Design review of the part built by this model. Coordinates are the model's own, in mm. A direction names the side the tool comes from. Round coordinates to 2 decimals unless told otherwise and drop trailing zeros. Order: outer loops, then holes, each group sorted by start corner. A loop starts at its lowest first (then second) coordinate and runs counter-clockwise, first axis right, second up. Notation, with made-up numbers: (-7.5, -17.75) - (14.5, -17.75) arc R25 ccw to (14.5, 10.25) - close; hole circle Ø8 at (9, 65). An arc over 180 degrees is marked (long way). Write item = value, one per line.
Autodesk Inventor part; units mm, degrees
ref_plane "YZ Plane" through (0, 0, 0) normal (1, 0, 0) x (0, 1, 0)
ref_plane "XZ Plane" through (0, 0, 0) normal (0, 1, 0) x (-1, 0, 0)
ref_plane "XY Plane" through (0, 0, 0) normal (0, 0, 1) x (1, 0, 0)
sketch "Boceto1" plane through (0, 0, 0) normal (0, 1, 0) x (-1, 0, 0)
  line L0 (100, 80) -> (-100, 80)
  line L1 (-100, 80) -> (-100, -80)
  line L2 (-100, -80) -> (100, -80)
  line L3 (100, -80) -> (100, 80)
  line L4 (100, 80) -> (-100, -80) construction
  line L5 (-100, 80) -> (100, -80) construction
  point P0 (0, 0)
  dimension "d0" = 200
  dimension "d1" = 160
extrude "Extrusión1" add sketch "Boceto1" along normal blind 20
sketch "Boceto2" plane through (0, 20, 0) normal (0, 1, 0) x (1, 0, 0)
  line L0 (-100, 80) -> (-100, -80)
  line L1 (-100, 80) -> (-70, 80)
  line L2 (-70, 80) -> (-70, 40)
  line L3 (-70, 40) -> (-100, 40)
  line L4 (-100, 40) -> (-100, 80)
  line L5 (100, 80) -> (-100, 80)
  line L6 (0, 80) -> (0, 40)
  line L7 (100, 80) -> (70, 80)
  line L8 (70, 80) -> (70, 40)
  line L9 (70, 40) -> (100, 40)
  line L10 (100, 40) -> (100, 80)
  point P0 (0, 0)
  dimension "d4" = 30
  dimension "d5" = 40
extrude "Extrusión2" cut sketch "Boceto2" against normal blind 10
sketch "Boceto3" plane through (0, 20, 0) normal (0, 1, 0) x (1, 0, 0)
  line L0 (-70, 80) -> (-70, 40)
  line L1 (-70, 80.0001) -> (-70, 40)
  line L2 (-70, 40) -> (-100, 40)
  line L3 (-100, 40) -> (-100, 80.0001)
  line L4 (-100, 40) -> (-70, 40)
  line L5 (-70, 40) -> (-70, 80)
  line L6 (-70, 80) -> (-100, 80)
  line L7 (-100, 80) -> (-100, 40)
  circle A0 centre (-88.25, 58.25) radius 1.75
  circle A1 centre (-81.75, 51.75) radius 1.75
  line L8 (100, 80) -> (-100, 80)
  line L9 (0, 80) -> (0, 56.5)
  circle A2 centre (88.25, 58.25) radius 1.75
  circle A3 centre (81.75, 51.75) radius 1.75
  point P0 (0, 0)
  point P1 (-64.3507, 80)
  point P2 (-74.3507, 0)
  point P3 (-85, 80)
  dimension "d23" = 21.75
  dimension "d24" = 11.75
  dimension "d26" = 11.75
hole "Agujero1" at (-81.75, 20, -51.75) at (-88.25, 20, -58.25) at (81.75, 20, -51.75) at (88.25, 20, -58.25) direction (0, -1, 0) diameter 3.5 end through all
sketch "Boceto4" plane through (-100, 0, 80) normal (0, 0, 1) x (1, 0, 0)
  line L0 (30, 20) -> (60, 20)
  line L1 (60, 20) -> (60, 10)
  line L2 (60, 10) -> (30, 10)
  line L3 (30, 10) -> (30, 20)
  line L4 (0, 0) -> (0, 20)
  line L5 (100, 0) -> (100, 10)
  line L6 (170, 20) -> (140, 20)
  line L7 (140, 20) -> (140, 10)
  line L8 (140, 10) -> (170, 10)
  line L9 (170, 10) -> (170, 20)
  dimension "d34" = 30
  dimension "d35" = 10
  dimension "d36" = 30
extrude "Extrusión3" add sketch "Boceto4" along normal blind 40
sketch "Boceto5" plane through (0, 20, 0) normal (0, 1, 0) x (1, 0, 0)
  line L0 (59.9999, -50) -> (69.9999, -50)
  line L1 (49.9999, -101.75) -> (49.9999, -79.9497)
  line L2 (59.9999, -108.25) -> (59.9999, -50)
  line L3 (40, -80) -> (69.9999, -80)
  line L4 (49.9999, -79.9497) -> (40, -80)
  circle A0 centre (51.7499, -101.75) radius 1.75
  circle A1 centre (58.2499, -108.25) radius 1.75
  line L5 (69.9999, -80) -> (69.9999, -120)
  line L6 (40, -120) -> (40, -80)
  line L7 (69.9999, -120) -> (40, -120)
  line L8 (0, -50) -> (0, -71.75)
  line L9 (-40, -120) -> (-40, -80)
  line L10 (-49.9999, -101.75) -> (-49.9999, -79.9497)
  circle A2 centre (-51.7499, -101.75) radius 1.75
  circle A3 centre (-58.2499, -108.25) radius 1.75
  line L11 (-40, -80) -> (-69.9999, -80)
  line L12 (-69.9999, -120) -> (-40, -120)
  line L13 (-69.9999, -80) -> (-69.9999, -120)
  line L14 (-59.9999, -108.25) -> (-59.9999, -50)
  line L15 (-40, -120) -> (-69.9999, -120)
  line L16 (-69.9999, -80) -> (-69.9999, -120)
  line L17 (-40, -120) -> (-70, -120)
  line L18 (-40, -80) -> (-40, -120)
  line L19 (-59.9999, -110) -> (-49.9999, -110)
  line L20 (-49.9999, -110) -> (-49.9999, -100)
  line L21 (-49.9999, -100) -> (-59.9999, -100)
  line L22 (-59.9999, -100) -> (-59.9999, -110)
  line L23 (-100, 40) -> (-100, -80)
  point P0 (0, 0)
  point P1 (-56.75, -68.25)
  point P2 (-63.25, -61.75)
  point P3 (63.25, -61.75)
  point P4 (56.75, -68.25)
  dimension "d45" = 3.5
  dimension "d46" = 3.5
  dimension "d39" = 10
  dimension "d40" = 10
  dimension "d41" = 40
  dimension "d42" = 0
  dimension "d43" = 6.5
  dimension "d44" = 6.5
  dimension "d47" = 11.7499
  dimension "d48" = 11.75
  dimension "d49" = 0
  dimension "d50" = 11.75
  dimension "d51" = 0
  dimension "d97" = 40.0001
hole "Agujero2" at (-58.2499, 20, 108.25) at (-51.7499, 20, 101.75) at (51.7499, 20, 101.75) at (58.2499, 20, 108.25) direction (0, -1, 0) diameter 3.5 end through all
sketch "Boceto6" plane through (0, 20, 0) normal (0, 1, 0) x (1, 0, 0)
  circle A0 centre (-60.569, -13.1067) radius 10
  circle A1 centre (-29.569, -59.1067) radius 3.5
  line L0 (-60.569, -13.1067) -> (-39.0083, -13.1067)
  circle A2 centre (-29.569, 25.8933) radius 3.5
  circle A3 centre (-88.569, 25.8933) radius 3.5
  circle A4 centre (-88.569, -59.1067) radius 3.5
  line L1 (70.4544, -63.0517) -> (18.4544, -63.0517)
  line L2 (18.4544, -63.0517) -> (18.4544, 6.9483)
  line L3 (18.4544, 6.9483) -> (70.4544, 6.9483)
  line L4 (70.4544, 6.9483) -> (70.4544, -63.0517)
  line L5 (70.4544, 6.9483) -> (48.4544, 6.9483)
  line L6 (48.4544, 6.9483) -> (48.4544, 48.9483)
  line L7 (48.4544, 48.9483) -> (70.4544, 48.9483)
  line L8 (70.4544, 48.9483) -> (70.4544, 6.9483)
  line L9 (77.2288, -8.158) -> (77.2281, -5.6604)
  circle A5 centre (63.7706, -5.7606) radius 1.75
  line L10 (70.7641, -24.1464) -> (70.7641, 22.2796)
  circle A6 centre (35.8307, -5.7609) radius 1.75
  line L11 (25.1581, -13.2381) -> (25.1581, -10.7404)
  circle A7 centre (68.8507, -57.8309) radius 1.75
  line L12 (26.4277, 35.0051) -> (26.4277, 37.5029)
  circle A8 centre (20.6074, -56.5614) radius 1.75
  line L13 (18.6941, -55.9176) -> (70.7641, -55.9176)
  line L14 (18.6941, -55.9176) -> (18.6941, -7.6743)
  line L15 (44.7291, -55.9176) -> (44.7291, -31.7959)
  line L16 (63.7706, -28.0517) -> (26.4277, -28.0517)
  line L17 (44.7291, -23.5247) -> (44.7291, -31.7959)
  point P0 (0, 0)
  point P1 (-60.569, -16.6067)
  point P2 (45.425, 12.8886)
  point P3 (44.7291, -28.0517)
  dimension "d59" = 7
  dimension "d60" = 7
  dimension "d61" = 7
  dimension "d62" = 39
  dimension "d63" = 46
  dimension "d64" = 59
  dimension "d65" = 46
  dimension "d66" = 39
  dimension "d67" = 59
  dimension "d68" = 52
  dimension "d69" = 70
  dimension "d70" = 22
  dimension "d71" = 42
  dimension "d72" = 3.5
  dimension "d73" = 3.5
  dimension "d74" = 3.5
  dimension "d75" = 3.5
  dimension "d142" = 17.3763
  dimension "d143" = 12.7092
  dimension "d144" = 6.6837
  dimension "d145" = 12.7089
  dimension "d146" = 5.2208
  dimension "d147" = 1.6037
  dimension "d148" = 2.1531
  dimension "d149" = 6.4903
hole "Agujero3" at (68.8507, 20, 57.8309) at (20.6074, 20, 56.5614) at (63.7706, 20, 5.7606) at (35.8307, 20, 5.7609) direction (0, -1, 0) diameter 3.5 end through all
sketch "Boceto7" plane through (0, 20, 0) normal (0, 1, 0) x (1, 0, 0)
  circle A0 centre (-60.569, -13.1067) radius 10
  circle A1 centre (-29.569, -59.1067) radius 3.5
  line L0 (-60.569, -13.1067) -> (-39.0083, -13.1067)
  circle A2 centre (-29.569, 25.8933) radius 3.5
  circle A3 centre (-88.569, 25.8933) radius 3.5
  circle A4 centre (-88.569, -59.1067) radius 3.5
  point P0 (0, 0)
  point P1 (-60.569, -16.6067)
  dimension "d83" = 7
  dimension "d84" = 7
  dimension "d85" = 7
  dimension "d86" = 39
  dimension "d87" = 46
  dimension "d88" = 59
  dimension "d89" = 46
  dimension "d90" = 39
  dimension "d91" = 59
extrude "Extrusión4" cut sketch "Boceto7" against normal blind 20
ref_plane "Plano de trabajo1" through (0, 0, -80) normal (-1, 0, 0) x (0, 0, 1)
ref_plane "Plano de trabajo2" through (100, 0, 0) normal (0, 0, -1) x (-1, 0, 0)
sketch "Boceto8" plane through (0, 20, 0) normal (0, 1, 0) x (1, 0, 0)
  line L0 (80, -15) -> (90, -15)
  circle A0 centre (85, -10) radius 1.75
  line L1 (85, 10) -> (85, -10)
  line L2 (90, -15) -> (90, 15)
  circle A1 centre (85, 10) radius 1.75
  line L3 (80, 15) -> (80, -15)
  line L4 (90, 15) -> (80, -15) construction
  line L5 (80, 15) -> (90, -15) construction
  line L6 (90, 15) -> (80, 15)
  line L7 (100, -80) -> (100, 40)
  line L8 (0, 0) -> (20, -20)
  line L9 (0, 0) -> (28.2843, 0) construction
  line L10 (15, -60) -> (15, -70)
  circle A2 centre (10, -65) radius 1.75
  line L11 (-10, -65) -> (10, -65)
  line L12 (15, -70) -> (-15, -70)
  circle A3 centre (-10, -65) radius 1.75
  line L13 (-15, -60) -> (15, -60)
  line L14 (-15, -70) -> (15, -60) construction
  line L15 (-15, -60) -> (15, -70) construction
  line L16 (-15, -70) -> (-15, -60)
  line L17 (0, 0) -> (18.6615, 18.6615)
  line L18 (0, 0) -> (26.3913, 0) construction
  line L19 (-15, 60) -> (-15, 70)
  circle A4 centre (-10, 65) radius 1.75
  line L20 (10, 65) -> (-10, 65)
  line L21 (-15, 70) -> (15, 70)
  circle A5 centre (10, 65) radius 1.75
  line L22 (15, 60) -> (-15, 60)
  line L23 (15, 70) -> (-15, 60) construction
  line L24 (15, 60) -> (-15, 70) construction
  line L25 (15, 70) -> (15, 60)
  line L26 (70, 80) -> (-70, 80)
  line L27 (-40, -80) -> (40, -80)
  point P0 (86.9608, 0)
  point P1 (86.9608, 0)
  point P2 (85, 15)
  point P3 (0, -69.1269)
  point P4 (0, -69.1269)
  point P5 (-15, -67.1661)
  point P6 (0, 69.7066)
  point P7 (0, 69.7066)
  point P8 (15, 67.7458)
  point P9 (-15, 65)
  point P10 (15, -65)
  dimension "d98" = 10
  dimension "d99" = 30
  dimension "d100" = 10
  dimension "d101" = 5
  dimension "d102" = 5
  dimension "d103" = 5
  dimension "d104" = 5
  dimension "d105" = 45
  dimension "d106" = 45
  dimension "d107" = 10
  dimension "d108" = 10
  dimension "d109" = 30
  dimension "d110" = 5
  dimension "d111" = 5
  dimension "d112" = 5
  dimension "d113" = 5
  dimension "d114" = 10
  dimension "d115" = 30
  dimension "d116" = 5
  dimension "d117" = 5
  dimension "d118" = 5
  dimension "d119" = 5
  dimension "d120" = 10
hole "Agujero4" at (-10, 20, -65) at (10, 20, -65) at (85, 20, -10) at (85, 20, 10) at (10, 20, 65) at (-10, 20, 65) direction (0, -1, 0) diameter 3.5 end through all
sketch "Boceto9" plane through (0, 20, 0) normal (0, 1, 0) x (1, 0, 0)
  circle A0 centre (10, -10) radius 1.75
  line L0 (6.803, 0) -> (14.6069, 0)
  line L1 (0, 0) -> (0, -4.8284)
  line L2 (0, 0) -> (20.0354, 0)
  circle A1 centre (10, 10) radius 1.75
  line L3 (0, 0) -> (0, 4.8284)
  circle A2 centre (-10, 10) radius 1.75
  circle A3 centre (-10, -10) radius 1.75
  dimension "d128" = 3.5
  dimension "d129" = 10
  dimension "d130" = 10
hole "Agujero5" at (-10, 20, 10) at (-10, 20, -10) at (10, 20, -10) at (10, 20, 10) direction (0, -1, 0) diameter 3.5 end through all
sketch "Boceto10" plane through (0, 0, 0) normal (0, -1, 0) x (1, 0, 0)
  line L0 (-16, 16) -> (16, 16)
  line L1 (16, 16) -> (16, -16)
  line L2 (16, -16) -> (-16, -16)
  line L3 (-16, -16) -> (-16, 16)
  line L4 (-16, 16) -> (16, -16) construction
  line L5 (16, 16) -> (-16, -16) construction
  point P0 (0, 0)
  point P1 (0, 0)
  dimension "d138" = 32
  dimension "d139" = 32
extrude "Extrusión5" cut sketch "Boceto10" against normal blind 10
sketch "Boceto11" plane through (0, 0, 0) normal (0, -1, 0) x (1, 0, 0)
  circle A0 centre (-88.569, 59.1067) radius 3.5
  circle A1 centre (-29.569, 59.1067) radius 3.5
  line L0 (-88.569, 59.1067) -> (-29.569, 59.1067)
  circle A2 centre (-29.569, -25.8933) radius 3.5
  line L1 (-29.569, 59.1067) -> (-29.569, -25.8933)
  circle A3 centre (-88.569, -25.8933) radius 3.5
  line L2 (-29.569, -25.8933) -> (-88.569, -25.8933)
  line L3 (-88.569, -25.8933) -> (-88.569, 59.1067)
  line L4 (-96.569, 66.6067) -> (-21.569, 66.6067)
  line L5 (-21.569, 66.6067) -> (-21.569, 51.6067)
  line L6 (-21.569, 51.6067) -> (-80.569, 51.6067)
  line L7 (-96.569, 51.6067) -> (-96.569, 66.6067)
  line L8 (-96.569, 66.6067) -> (-21.569, 51.6067) construction
  line L9 (-21.569, 66.6067) -> (-96.569, 51.6067) construction
  line L10 (-37.569, -33.3933) -> (-21.569, -33.3933)
  line L11 (-21.569, -33.3933) -> (-21.569, 66.6067)
  line L12 (-21.569, 66.6067) -> (-37.569, 66.6067)
  line L13 (-37.569, 66.6067) -> (-37.569, 51.6067)
  line L14 (-37.569, -33.3933) -> (-21.569, 66.6067) construction
  line L15 (-21.569, -33.3933) -> (-37.569, 66.6067) construction
  line L16 (-96.569, -18.3933) -> (-80.569, -18.3933)
  line L17 (-21.569, -18.3933) -> (-21.569, -33.3933)
  line L18 (-21.569, -33.3933) -> (-96.569, -33.3933)
  line L19 (-96.569, -33.3933) -> (-96.569, -18.3933)
  line L20 (-96.569, -18.3933) -> (-21.569, -33.3933) construction
  line L21 (-21.569, -18.3933) -> (-96.569, -33.3933) construction
  line L22 (-80.569, -33.3933) -> (-96.569, -33.3933)
  line L23 (-96.569, -33.3933) -> (-96.569, 66.6067)
  line L24 (-96.569, 66.6067) -> (-80.569, 66.6067)
  line L25 (-80.569, 66.6067) -> (-80.569, 51.6067)
  line L26 (-80.569, -33.3933) -> (-96.569, 66.6067) construction
  line L27 (-96.569, -33.3933) -> (-80.569, 66.6067) construction
  line L28 (-80.569, -18.3933) -> (-37.569, -18.3933)
  line L29 (-80.569, 51.6067) -> (-96.569, 51.6067)
  line L30 (-80.569, 51.6067) -> (-80.569, -33.3933)
  line L31 (-37.569, -18.3933) -> (-21.569, -18.3933)
  line L32 (-37.569, -18.3933) -> (-37.569, -33.3933)
  line L33 (-37.569, 51.6067) -> (-37.569, -18.3933)
  circle A4 centre (-88.569, 59.1067) radius 3.5
  circle A5 centre (-29.569, 59.1067) radius 3.5
  circle A6 centre (-29.569, -25.8933) radius 3.5
  circle A7 centre (-88.569, -25.8933) radius 3.5
  point P0 (0, 0)
  point P1 (-59.069, 59.1067)
  point P2 (-29.569, 16.6067)
  point P3 (-59.069, -25.8933)
  point P4 (-88.569, 16.6067)
  dimension "d150" = 75
  dimension "d151" = 15
properties part number "base_mid_20"
Item 1: For line 1 along X through (y, z) = (15, -10); line 2 along Z through (x, y) = (88.25, 3.5); line 3 along Z through (x, y) = (85, 14), list the stretches that pass through material, from the lowest coordinate up. Write a range as [from, to].
Data:
line_1 = [-100, -11.75], [-8.25, 8.25], [11.75, 83.25], [86.75, 100]
line_2 = [-80, -60], [-56.5, 80]
line_3 = [-40, -11.75], [-8.25, 8.25], [11.75, 80]
Item 2: Insertion check: P1, Ø11, axis at y = 16.5, z = 100.5, coming from the -X side; P2, Ø9, axis at x = 88.5, z = -67, coming from the +Y side; P3, Ø8, axis at y = 13.5, z = 99.5, coming from the +X side. Each pin has a flat end and moves straight along its axis. Give the tip position at first contact, or say it passes through.
Data:
P1 = -70
P2 = 10
P3 = 70
Item 3: Take a section at B-B, the plane y = 2.5. Count the separate pieces of the cut face and the enclosed holes in it, and give its area (3 significant figures).
Data:
separate_pieces = 1
enclosed_holes = 20
area = 30,400 mm2
Item 4: For faces 1 (the face through (40, 15, 100)), 2 (the face through (-85, 10, -60)), 3 (the face through (-55, 10, 100)), 4 (the face through (16, 5, 0)), 5 (the face through (85, 10, -60)), list the 3-axis set-ups (+Z, -Z, +X, -X, +Y, -Y) from which the entire face can be reached by the end or side of a thin tool; tool diameter is ignored.
Data:
face_1 = +Z, +Y, -Y
face_2 = -Z, -X, +Y
face_3 = +Z, +X, -X, -Y
face_4 = -Y
face_5 = -Z, +X, +Y
Item 5: The part is to be moulded in two halves that separate along X. For faces 6 (the face through (-55, 15, 120)), 7 (the face through (-100, 10, -1)), 8 (the face through (0, 5, -16)), say which applies: +X half, -X half, draft (parallel to the pull), parting line (faces both ways), or undercut.
Data:
face_6 = draft
face_7 = -X half
face_8 = undercut
Item 6: Take a section at C-C, the plane x = 4. State the section outline as (y, z) points, and give its area (3 significant figures).
Data:
outline = (0, -80) - (20, -80) - (20, 80) - (0, 80) - (0, 16) - (10, 16) - (10, -16) - (0, -16) - close
area = 2,880 mm2
Item 7: Take a section at A-A, the plane z = 19.5. State the section outline as (x, y) points.
Data:
outline = (-100, 0) - (-68.26, 0) - (-68.26, 20) - (-100, 20) - close; (-52.88, 0) - (100, 0) - (100, 20) - (-52.88, 20) - close
